Design review of the part built by this model. Coordinates are the model's own, in mm. Coordinates: 2 decimals unless noted, no trailing zeros. Write each loop counter-clockwise with the first axis right and the second up, starting at its lowest first coordinate (ties: lowest second). Pieces come first, ordered by that corner, then holes.
Q1. The part is to be moulded in two halves that separate along X. For faces 1 (the face through (-0.2, 1, -7.5)), 2 (the face through (15, 1, -2)), 3 (the face through (-15, 1, -2)), 4 (the face through (0, 0, 0)), say which applies: +X half, -X half, draft (parallel to the pull), parting line (faces both ways), or undercut.
Q2. Add section B-B, the plane x = 1. Give the boundary of the cut face in (y, z), plus the area to 3 significant figures.
Q3. To check wall thickness, follow probe 1 along Y at (x, z) = (-0.5, -7.25); probe 2 along X at (y, z) = (0.9, -9.75); probe 3 along Z at (x, y) = (-11.75, 0.7). State the ranges of each line that lie inside material, in increasing order.
Q4. Add section A-A, the plane z = -8. Give the boundary of the cut face in (x, y).
Q5. Add section C-C, the plane y = 0.6. Give the boundary of the cut face in (x, z).
Q6. Add section D-D, the plane x = -12. Give the boundary of the cut face in (y, z), plus the area to 3 significant figures.
Q7. Clearance check with flat-ended pins moving along their axes: pin 1 Ø6 at (x, z) = (8.5, -5.5) entering from -Y; pin 2 Ø1 at (x, y) = (-10, 1.5) entering from -Z. State where each tip first meets the part, or that it passes through.
from build123d import *

# Parameters (mm, degrees)
SKETCH1_W           = 30
SKETCH1_H           = 25
BOSS_EXTRUDE1_DEPTH = 2
SKETCH2_W           = 30
SKETCH2_H           = 2
BOSS_EXTRUDE2_DEPTH = 12.5
CUT_EXTRUDE1_REACH  = 25.184
SKETCH3_R           = 25
FILLET1_R           = 2
CUT_EXTRUDE2_REACH  = 26.321
SKETCH4_W           = 35.566243018
SKETCH4_H           = 17.679126646


with BuildPart() as part:
    # Sketch1 → Boss-Extrude1 (new body)
    with BuildSketch(Plane(origin=(0, 0, 0), x_dir=(1, 0, 0), z_dir=(0, 1, 0))):
        Rectangle(SKETCH1_W, SKETCH1_H)
    extrude(amount=BOSS_EXTRUDE1_DEPTH)

    # Sketch2 → Boss-Extrude2 (add)
    with BuildSketch(Plane(origin=(0, 0, 0), x_dir=(1, 0, 0), z_dir=(0, 1, 0))):
        with Locations((0, -11.5)):
            Rectangle(SKETCH2_W, SKETCH2_H)
    extrude(amount=-BOSS_EXTRUDE2_DEPTH)

    # Sketch3 → Cut-Extrude1 (cut, up to next)
    with BuildSketch(Plane(origin=(0, 0, 0), x_dir=(1, 0, 0), z_dir=(0, 1, 0)), mode=Mode.PRIVATE) as cut_extrude1_sk1:
        with Locations((0, 32.5)):
            Circle(SKETCH3_R)
    cut_extrude1_tool1 = extrude(cut_extrude1_sk1.sketch, amount=CUT_EXTRUDE1_REACH, mode=Mode.PRIVATE) & part.part
    add(cut_extrude1_tool1.solids().sort_by_distance((0, 0, -32.5))[0], mode=Mode.SUBTRACT)

    # Fillet1
    fillet1_edges = [part.edges().sort_by_distance(p)[0] for p in [
        (0, 0, 10.5),
    ]]
    fillet(fillet1_edges, radius=FILLET1_R)

    # Sketch4 → Cut-Extrude2 (cut, up to next)
    with BuildSketch(Plane(origin=(0, 2, 0), x_dir=(1, 0, 0), z_dir=(0, 1, 0)), mode=Mode.PRIVATE) as cut_extrude2_sk1:
        with Locations((0, -17.523134352)):
            Rectangle(SKETCH4_W, SKETCH4_H)
    cut_extrude2_tool1 = extrude(cut_extrude2_sk1.sketch, amount=-CUT_EXTRUDE2_REACH, mode=Mode.PRIVATE) & part.part
    add(cut_extrude2_tool1.solids().sort_by_distance((0, 2, 17.523134))[0], mode=Mode.SUBTRACT)


solid = part.part
Here are the results:
1. face 1: undercut
1. face 2: +X half
1. face 3: -X half
1. face 4: draft
2. outline: (-0.01, 8.68) arc R2 cw to (0, 8.5) - (0, -7.52) - (2, -7.52) - (2, 8.68) - close
2. area: 32.4 mm2
3. probe 1: y = 0 to 2
3. probe 2: x = -15 to -10.37, 10.37 to 15
3. probe 3: z = -10.43 to 8.68
4. outline: (-15, 0) - (-4.97, 0) - (-4.97, 2) - (-15, 2) - close; (4.97, 0) - (15, 0) - (15, 2) - (4.97, 2) - close
5. outline: (-15, -12.5) arc R25 cw to (15, -12.5) - (15, 8.68) - (-15, 8.68) - close
6. outline: (-0.01, 8.68) arc R2 cw to (0, 8.5) - (0, -10.57) - (2, -10.57) - (2, 8.68) - close
6. area: 38.5 mm2
7. pin 1: stops at y = 0
7. pin 2: stops at z = -9.81
